Design review of the part built by this model. Coordinates are the model's own, in mm. A direction names the side the tool comes from. Give positions to 0.01 mm unless a question says otherwise; leave off trailing zeros. Loops run counter-clockwise (first coordinate to the right, second up) from the corner with the lowest first, then second, coordinate; pieces in that order, holes last. Notation, with made-up numbers: M 51.5,-20 L 97.5,-20 A17 ccw 97.5,2 Z; hole C -35,78 d7. An arc over 180 degrees is marked long. Answer as CSV lines item,"result".
```python
from build123d import *

# Parameters (mm, degrees)
SKETCH_2_R          = 1.75
CUT_EXTRUDE_1_DEPTH = 22.610182785


with BuildPart() as part:
    # 草图1 → 旋转1 (revolve)
    with BuildSketch(Plane(origin=(0, 0, 0), x_dir=(1, 0, 0), z_dir=(0, 1, 0)), mode=Mode.PRIVATE) as revolve_1_sk:
        Polygon((4, 15), (4, 0), (5.1, 0), (5.1, 11.5), (11, 11.5), (11, 15), align=None)
    revolve(revolve_1_sk.sketch.rotate(Axis((0, 0, -35.917436649), (0, 0, 1)), 180), axis=Axis((0, 0, -35.917436649), (0, 0, 1)))

    # 草图2 → 切除-拉伸1 (cut, through all)
    with BuildSketch(Plane(origin=(0, 0, -15), x_dir=(-1, 0, 0), z_dir=(0, 0, -1))):
        with Locations((0, 8)):
            Circle(SKETCH_2_R)
        with Locations((8, 0)):
            Circle(SKETCH_2_R)
        with Locations((0, -8)):
            Circle(SKETCH_2_R)
        with Locations((-8, 0)):
            Circle(SKETCH_2_R)
    extrude(amount=-CUT_EXTRUDE_1_DEPTH, mode=Mode.SUBTRACT)


solid = part.part
```
1. We need section C-C, the plane y = -8.5. Write out the cut boundary in (x, z).
Answer block:
outline,"M -6.98,-15 L -1.68,-15 L -1.68,-11.5 L -6.98,-11.5 Z; M 1.68,-15 L 6.98,-15 L 6.98,-11.5 L 1.68,-11.5 Z"
2. The part is to be moulded in two halves that separate along X. For faces 3 (the flat face through (0, 5, -15)), 4 (the cylindrical face through (-1.617, -8.67, -13.274)), 5 (the cylindrical face through (-4.864, -1.532, -5.83)), say which applies: pulls with the +X half, pulls with the -X half, needs draft (parallel to the pull), parting line crosses it, or undercut.
Answer block:
face 3,"needs draft"
face 4,"undercut"
face 5,"parting line crosses it"
3. For faces 1 (the cylindrical face through (-9.669, 0.526, -13.274)), 2 (the flat face through (2, 5, -11.5)), list the 3-axis set-ups (+Z, -Z, +X, -X, +Y, -Y) from which the entire face can be reached by the end or side of a thin tool; tool diameter is ignored.
Answer block:
face 1,"+Z, -Z"
face 2,"+Z"
4. We need section A-A, the plane x = 0. Write out the cut boundary in (y, z).
Answer block:
outline,"M -11,-15 L -9.75,-15 L -9.75,-11.5 L -11,-11.5 Z; M -6.25,-15 L -4,-15 L -4,0 L -5.1,0 L -5.1,-11.5 L -6.25,-11.5 Z; M 4,-15 L 6.25,-15 L 6.25,-11.5 L 5.1,-11.5 L 5.1,0 L 4,0 Z; M 9.75,-15 L 11,-15 L 11,-11.5 L 9.75,-11.5 Z"
5. For P1, Ø8, axis at y = -4.5, z = -2, coming from the +X side; P2, Ø4, axis at x = 8.5, y = -7.5, coming from the +Z side; P3, Ø2, axis at x = -2.5, z = -3.5, coming from the +Y side, all flat-tipped, find the tip position at first contact; note any pin that passes through.
Answer block:
P1,"x = 5.08"
P2,"z = -11.5"
P3,"y = 4.87"
6. To check wall thickness, follow L1, parallel to Y at x = 0, z = -13.6; L2, parallel to Z at x = 8, y = 3.25; L3, parallel to Y at x = 9, z = -12. State the ranges of each line that lie inside material, in increasing order. Write a range as [from, to].
Answer block:
L1,"[-11, -9.75], [-6.25, -4], [4, 6.25], [9.75, 11]"
L2,"[-15, -11.5]"
L3,"[-6.32, -1.44], [1.44, 6.32]"
7. We need section B-B, the plane x = -8. Write out the cut boundary in (y, z).
Answer block:
outline,"M -7.55,-15 L -1.75,-15 L -1.75,-11.5 L -7.55,-11.5 Z; M 1.75,-15 L 7.55,-15 L 7.55,-11.5 L 1.75,-11.5 Z"
8. We need section D-D, the plane z = -12. Write out the cut boundary in (x, y).
Answer block:
outline,"C 0,0 d22; hole C -8,0 d3.5; hole C 0,0 d8; hole C 0,-8 d3.5; hole C 0,8 d3.5; hole C 8,0 d3.5"
